Design review of the part built by this model. Coordinates are the model's own, in mm. A direction names the side the tool comes from. Round coordinates to 2 decimals unless told otherwise and drop trailing zeros. Order: outer loops, then holes, each group sorted by start corner. A loop starts at its lowest first (then second) coordinate and runs counter-clockwise, first axis right, second up. Notation, with made-up numbers: (43, -7) - (91, -7) arc R29 cw to (91, 23) - close; hole circle Ø9 at (82.25, 19). An arc over 180 degrees is marked (long way). Write item = value, one per line.
from build123d import *

# Parameters (mm, degrees)
SKETCH004_W  = 56
SKETCH004_H  = 53.6
PAD002_DEPTH = 1.2
FILLET002_R  = 2
FILLET003_R  = 0.5
PAD003_DEPTH = 3
FILLET004_R  = 1


with BuildPart() as part:
    # Sketch004 → Pad002 (new body)
    with BuildSketch(Plane.XY):
        Rectangle(SKETCH004_W, SKETCH004_H)
    extrude(amount=PAD002_DEPTH)

    # Fillet002
    fillet002_edges = [part.edges().sort_by_distance(p)[0] for p in [
        (-28, -26.8, 0.6),
        (-28, 26.8, 0.6),
        (28, -26.8, 0.6),
        (28, 26.8, 0.6),
    ]]
    fillet(fillet002_edges, radius=FILLET002_R)

    # Fillet003
    fillet003_edges = [part.edges().sort_by_distance(p)[0] for p in [
        (0, 26.8, 1.2),
        (-28, 0, 0),
    ]]
    fillet(fillet003_edges, radius=FILLET003_R)

    # Sketch005 (on Face9 of Fillet003) → Pad003 (join)
    with BuildSketch(Plane(origin=(0, 0, 0), x_dir=(1, 0, 0), z_dir=(0, 0, -1))):
        with BuildLine():
            ThreePointArc((1.5, 2), (0, 3.5), (-1.5, 2))
            Line((-1.5, 2), (-1.5, -2))
            ThreePointArc((-1.5, -2), (0, -3.5), (1.5, -2))
            Line((1.5, -2), (1.5, 2))
        make_face()
    extrude(amount=PAD003_DEPTH)

    # Fillet004
    fillet004_edges = [part.edges().sort_by_distance(p)[0] for p in [
        (-1.5, 0, -3),
    ]]
    fillet(fillet004_edges, radius=FILLET004_R)


solid = part.part
Item 1: Take a section at C-C, the plane z = -0.85. State the section outline as (x, y) points.
Data:
outline = (-1.5, -2) arc R1.5 ccw to (1.5, -2) - (1.5, 2) arc R1.5 ccw to (-1.5, 2) - close
Item 2: Insertion check: P1, Ø1.5, axis at x = -3, z = -0.5, coming from the +Y side; P2, Ø5, axis at x = -10, y = 11.5, coming from the -Z side; P3, Ø1.5, axis at x = 11, z = -1.5, coming from the +Y side (3 decimals). Each pin has a flat end and moves straight along its axis. Give the tip position at first contact, or say it passes through.
Data:
P1 = 26.73
P2 = 0
P3 = through
Item 3: Take a section at B-B, the plane x = -9. State the section outline as (y, z) points, and give its area (3 significant figures).
Data:
outline = (-26.8, 0.5) arc R0.5 ccw to (-26.3, 0) - (26.3, 0) arc R0.5 ccw to (26.8, 0.5) - (26.8, 0.7) arc R0.5 ccw to (26.3, 1.2) - (-26.3, 1.2) arc R0.5 ccw to (-26.8, 0.7) - close
area = 64.1 mm2
Item 4: For faces 1 (the face through (-1.5, 0, -1)), 2 (the face through (0, 3.5, -1)), 3 (the face through (1.5, 0, -1)), list the 3-axis set-ups (+Z, -Z, +X, -X, +Y, -Y) from which the entire face can be reached by the end or side of a thin tool; tool diameter is ignored.
Data:
face_1 = -Z, -X, +Y, -Y
face_2 = -Z, +Y
face_3 = -Z, +X, +Y, -Y
Item 5: Take a section at A-A, the plane y = 23. State the section outline as (x, z) points.
Data:
outline = (-28, 0.5) arc R0.5 ccw to (-27.5, 0) - (27.5, 0) arc R0.5 ccw to (28, 0.5) - (28, 0.7) arc R0.5 ccw to (27.5, 1.2) - (-27.5, 1.2) arc R0.5 ccw to (-28, 0.7) - close
Item 6: For line 1 along Z through (x, y) = (-20.5, -2); line 2 along X through (y, z) = (-23, 0.95); line 3 along Y through (x, z) = (4, 0.45), list the stretches that pass through material, from the lowest coordinate up. Write a range as [from, to].
Data:
line_1 = [0, 1.2]
line_2 = [-27.93, 27.93]
line_3 = [-26.8, 26.8]
